from build123d import *

# Parameters (mm, degrees)
F0_W     = 76.2
F0_H     = 101.6
F1_DEPTH = 133.35
F3_DEPTH = 76.201
F4_W     = 34.9662494294
F4_H     = 12.1309220302
F5_DEPTH = 25.4
F6_W     = 20.8403859288
F6_H     = 113.2664903998
F7_DEPTH = 25.4


# Not quite as in the source:
# - a feature names something its author has since deleted; it is built from what else it names


with BuildPart() as f1:
    # F0 (on Top) → F1 (new body)
    with BuildSketch(Plane.XY):
        Rectangle(F0_W, F0_H)
    extrude(amount=F1_DEPTH)

    # F2 (on face) → F3 (cut, through all)
    with BuildSketch(Plane.YZ.offset(38.1)):
        with BuildLine():
            Line((49.114014449, 0), (50.8, 0))
            Line((50.8, 0), (50.8, 66.2650913))
            Line((50.8, 66.2650913), (50.8, 73.7310647964))
            Line((50.8, 73.7310647964), (50.8, 128.6014442141))
            Line((50.8, 128.6014442141), (50.8, 133.35))
            Line((50.8, 133.35), (-50.8, 133.35))
            Line((-50.8, 133.35), (-50.8, 0))
            Line((-50.8, 0), (-49.3153884285, 0))
            ThreePointArc((-49.3153884285, 0), (-49.8930613229, 0.38308634), (-49.7649416709, 1.0642959051))
            Line((-49.7649416709, 1.0642959051), (-42.2846688887, 8.7558660005))
            ThreePointArc((-42.2846688887, 8.7558660005), (-41.4521127702, 9.3248290153), (-40.4637807514, 9.525))
            Line((-40.4637807514, 9.525), (-38.2985454719, 9.525))
            ThreePointArc((-38.2985454719, 9.525), (-34.4105014329, 10.8544807489), (-32.1505139925, 14.2862240786))
            Line((-32.1505139925, 14.2862240786), (-26.0325690106, 37.9606251271))
            ThreePointArc((-26.0325690106, 37.9606251271), (-26.3063034957, 39.9399780989), (-27.8936985581, 41.1536278306))
            Line((-27.8936985581, 41.1536278306), (-38.7149990474, 44.0606170611))
            ThreePointArc((-38.7149990474, 44.0606170611), (-40.050293777, 44.9146793042), (-40.6508289049, 46.3815780362))
            Line((-40.6508289049, 46.3815780362), (-41.828178264, 60.7104246977))
            ThreePointArc((-41.828178264, 60.7104246977), (-41.1424179273, 62.7046091009), (-39.2110885015, 63.5513707689))
            Line((-39.2110885015, 63.5513707689), (-32.5366084985, 63.5513707689))
            Line((-32.5366084985, 63.5513707689), (-34.9197723805, 54.3293235498))
            Line((-34.9197723805, 54.3293235498), (-22.6237094217, 51.1517717071))
            Line((-22.6237094217, 51.1517717071), (-2.6091445634, 128.6014442141))
            Line((-2.6091445634, 128.6014442141), (6.5897179326, 126.1302999894))
            Line((6.5897179326, 126.1302999894), (-18.753958765, 28.0587468857))
            ThreePointArc((-18.753958765, 28.0587468857), (-17.3156963729, 20.1857452314), (-10.3820422123, 16.1885970308))
            Line((-10.3820422123, 16.1885970308), (32.5785662344, 12.338888515))
            ThreePointArc((32.5785662344, 12.338888515), (34.2472884437, 11.9577274025), (35.7535762689, 11.144699363))
            Line((35.7535762689, 11.144699363), (49.5238091926, 1.1017641769))
            ThreePointArc((49.5238091926, 1.1017641769), (49.7017678057, 0.4084810434), (49.114014449, 0))
        make_face()
    extrude(amount=-F3_DEPTH, mode=Mode.SUBTRACT)

    # F4 (on face) → F5 (cut)
    with BuildSketch(Plane(origin=(0, -33.598613666, 8.682562632), x_dir=(1, 0, 0), z_dir=(0, -0.9681939338, 0.2502009325))):
        Polygon((19.05, 73.9268932369), (-15.9162494294, 83.0707615279), (-15.9162494294, 43.8643618742), (19.05, 43.8643618742), align=None)
        with Locations((1.5668752853, 37.7989008591)):
            Rectangle(F4_W, F4_H)
    extrude(amount=F5_DEPTH, mode=Mode.SUBTRACT)

    # F6 (on face) → F7 (cut)
    with BuildSketch(Plane(origin=(0, 0, 0), x_dir=(1, 0, 0), z_dir=(0, 0, -1))):
        Rectangle(F6_W, F6_H)
    extrude(amount=-F7_DEPTH, mode=Mode.SUBTRACT)


solid = f1.part
Read the model definition and answer for the solid it produces. Units are mm, in the model's axes. A direction names the side the tool comes from. Coordinates: 2 decimals unless noted, no trailing zeros. Loops run counter-clockwise (first coordinate to the right, second up) from the corner with the lowest first, then second, coordinate; pieces in that order, holes last. Notation, with made-up numbers: (29.5, 36.25) - (74.5, 36.25) arc R20 cw to (74.5, 45.25) - close; hole circle Ø7 at (53.5, 41). An arc over 180 degrees is marked (long way). Answer in a Markdown table with one row per item.
Q1. Straight lines are drawn through the part: line 1 along Z through (x, y) = (15.5, 42); line 2 along Y through (x, z) = (26.5, 62); line 3 along Y through (x, z) = (9, 84.5). For each, find the intervals that lie inside material, in ascending order. Write a range as [from, to].
Here are the results:
| item | result |
|---|---|
| line 1 | z = [0, 6.59] |
| line 2 | y = [-41.61, -32.94], [-19.82, -9.98] |
| line 3 | y = [-14.01, -4.17] |
Q2. For faces 1 (the flat face through (0.5, -5.9, 77.8)), 2 (the flat face through (10.42, 1, 7)), 3 (the flat face through (28.708, -33.229, 42.587)), determine the directions among +Z, -Z, +X, -X, +Y, -Y from which every point of the face is accessible in a straight line to the end or side of a thin tool.
Here are the results:
| item | result |
|---|---|
| face 1 | +X, -X, +Y |
| face 2 | -Z, +Y, -Y |
| face 3 | +X, -X, -Y |
Q3. Find section C-C on y = 4.5. Write down the section's boundary in (x, z).
Here are the results:
| item | result |
|---|---|
| outline | (-38.1, 0) - (-10.42, 0) - (-10.42, 14.86) - (-38.1, 14.86) - close; (-38.1, 118.04) - (38.1, 118.04) - (38.1, 126.69) - (-38.1, 126.69) - close; (10.42, 0) - (38.1, 0) - (38.1, 14.86) - (10.42, 14.86) - close |
Q4. Find section B-B on y = 38. Write down the section's boundary in (x, z), plus the area to 3 significant figures.
Here are the results:
| item | result |
|---|---|
| outline | (-38.1, 0) - (-10.42, 0) - (-10.42, 9.51) - (-38.1, 9.51) - close; (10.42, 0) - (38.1, 0) - (38.1, 9.51) - (10.42, 9.51) - close |
| area | 526 mm^2 |
Q5. Given P1, Ø1.1, axis at x = 20, y = -40, coming from the +Z side; P2, Ø12, axis at y = 5.5, z = 83.5, coming from the -X side; P3, Ø2, axis at x = 32.5, y = -36.5, coming from the +Z side; P4, Ø3, axis at x = -2.5, y = -25.5, coming from the -Z side, each flat-ended and moving along its own axis, determine where each tip first touches the part or whether it passes through.
Here are the results:
| item | result |
|---|---|
| P1 | stops at z = 63.54 |
| P2 | passes through |
| P3 | stops at z = 63.55 |
| P4 | stops at z = 25.4 |
Q6. Find section D-D on x = 1.5. Write down the section's boundary in (y, z) (3 decimals), plus the area to 3 significant figures.
Here are the results:
| item | result |
|---|---|
| outline | (-29.278, 25.4) - (-19.053, 25.4) arc R9.525 cw to (-18.754, 28.059) - (6.59, 126.13) - (-2.609, 128.601) - (-25.659, 39.407) - (-26.11, 39.523) arc R2.626 cw to (-26.033, 37.961) - close |
| area | 1,000 mm^2 |
Q7. The mould has two halves that part along Y. Classify faces 4 (the cylindrical face through (24.45, 34.22, 11.97)), 5 (the flat face through (24, 1, 0)), 6 (the flat face through (-26.853, -33.712, 59.005)), 7 (the cylindrical face through (-24.066, -34.457, 10.819)): pulls with the +Y half, pulls with the -Y half, needs draft (parallel to the pull), parting line crosses it, or undercut.
Here are the results:
| item | result |
|---|---|
| face 4 | pulls with the +Y half |
| face 5 | needs draft |
| face 6 | undercut |
| face 7 | pulls with the -Y half |
Q8. Find section A-A on x = 30.5. Write down the section's boundary in (y, z) (3 decimals).
Here are the results:
| item | result |
|---|---|
| outline | (-49.765, 1.064) arc R0.627 ccw to (-49.315, 0) - (49.114, 0) arc R0.627 ccw to (49.524, 1.102) - (35.754, 11.145) arc R6.35 ccw to (32.579, 12.339) - (-10.382, 16.189) arc R9.525 cw to (-18.754, 28.059) - (6.59, 126.13) - (-2.609, 128.601) - (-22.624, 51.152) - (-34.92, 54.329) - (-32.537, 63.551) - (-39.211, 63.551) arc R2.626 ccw to (-41.828, 60.71) - (-40.651, 46.382) arc R2.626 ccw to (-38.715, 44.061) - (-27.894, 41.154) arc R2.626 cw to (-26.033, 37.961) - (-32.151, 14.286) arc R6.35 cw to (-38.299, 9.525) - (-40.464, 9.525) arc R2.54 ccw to (-42.285, 8.756) - close |
